The listing builds one solid part. Answer for the finished solid, in the listing's coordinates (mm). Face numbers are marked on the shaded views. Give positions to 0.01 mm unless a question says otherwise; leave off trailing zeros. Write each loop counter-clockwise with the first axis right and the second up, starting at its lowest first coordinate (ties: lowest second). Pieces come first, ordered by that corner, then holes. Notation, with made-up numbers: (27.25, -4.75) - (58.25, -4.75) arc R26 cw to (58.25, 32.25) - close; hole circle Ø2 at (68, -40). An arc over 180 degrees is marked (long way). One line per question, with ' | ' between items. Start each with the question number.
1. The mould has two halves that part along Y. Classify the marked faces 1, 2 and 3: +Y half, -Y half, draft (parallel to the pull), parting line (faces both ways), or undercut.
2. Find the intervals of material crossed by L1, parallel to Y at x = -7.15, z = 1.05; L2, parallel to X at y = 0, z = -2.9; L3, parallel to Z at x = 2, y = -1, in increasing order. Write a range as from..to.
3. A cutting plane is placed at A-A (y = 16.15). Determine the outline of the cut face in (x, z).
4. Given P1, Ø1, axis at x = 16.15, y = 0, coming from the +Z side (1 decimal); P2, Ø4.5, axis at x = -2, y = 1.5, coming from the +Z side; P3, Ø2.5, axis at x = 0, y = -7.15, coming from the +Z side; P4, Ø5, axis at x = 3, y = -12, coming from the -Z side, each flat-ended and moving along its own axis, determine where each tip first touches the part or whether it passes through.
5. A cutting plane is placed at C-C (z = -1.85). Determine the outline of the cut face in (x, y), then the cut area to 3 significant figures.
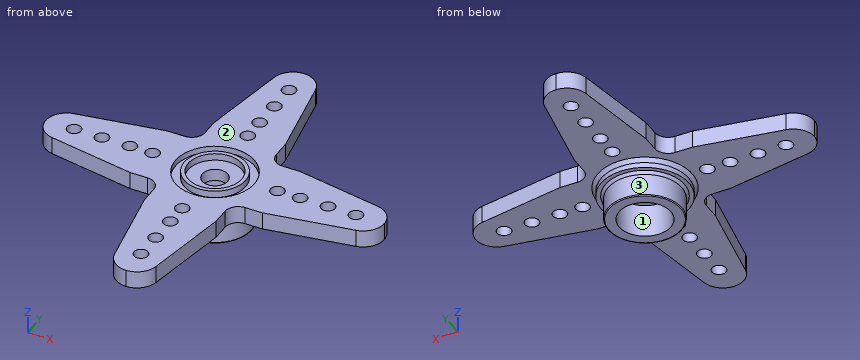
```python
from build123d import *

# Parameters (mm, degrees)
PAD_DEPTH          = 2
SKETCH001_R        = 4.5
POCKET_DEPTH       = 0.7
SKETCH002_R        = 3.5
PAD001_DEPTH       = 0.8
SKETCH003_R        = 3.05
POCKET001_DEPTH    = 0.8
SKETCH004_R        = 5
PAD002_DEPTH       = 1
SKETCH005_R        = 4.2
PAD003_DEPTH       = 2.9
SKETCH006_R        = 2.95
POCKET002_DEPTH    = 3.8
SKETCH007_R        = 1.45
POCKET003_DEPTH    = 5.201
SKETCH008_R        = 0.8
POCKET004_DEPTH    = 116.298101
POLARPATTERN_COUNT = 4
CHAMFER_SIZE       = 0.4
CHAMFER001_SIZE    = 0.3
FILLET_R           = 0.1


with BuildPart() as horn_top_left_quarter:
    # Sketch → Pad (new body)
    with BuildSketch(Plane.XY):
        with BuildLine():
            Line((0, 0), (0, 19.4))
            ThreePointArc((0, 19.4), (-1.543669, 18.837685), (-2.363981, 17.414237))
            Line((-4.086144, 7.586132), (-2.363981, 17.414237))
            Line((-4.086144, 5.586132), (-4.086144, 7.586132))
            ThreePointArc((-5.586136, 4.086144), (-4.525485, 4.525482), (-4.086144, 5.586132))
            Line((-5.586136, 4.086144), (-7.586136, 4.086144))
            Line((-17.414238, 2.363981), (-7.586136, 4.086144))
            ThreePointArc((-17.414238, 2.363981), (-18.837685, 1.543669), (-19.4, 0))
            Line((-19.4, 0), (0, 0))
        make_face()
    extrude(amount=PAD_DEPTH)


with BuildPart() as upper_half_horn:
    # Part__Mirroring: instance of horn-top-left-quarter
    add(horn_top_left_quarter.part.mirror(Plane(origin=(0, 0, 0), x_dir=(0, -1, 0), z_dir=(1, 0, 0))))

    # Fusion: union horn-top-left-quarter
    add(horn_top_left_quarter.part)


with BuildPart() as horn_final:
    # Part__Mirroring001: instance of Upper-half-horn
    add(upper_half_horn.part.mirror(Plane(origin=(0, 0, 0), x_dir=(1, 0, 0), z_dir=(0, 1, 0))))

    # Fusion001: union Upper-half-horn
    add(upper_half_horn.part)

    # Sketch001 (on Face24 of Fusion001) → Pocket (cut)
    with BuildSketch(Plane.XY.offset(2)):
        Circle(SKETCH001_R)
    extrude(amount=-POCKET_DEPTH, mode=Mode.SUBTRACT)

    # Sketch002 (on Face28 of Pocket) → Pad001 (new body)
    with BuildSketch(Plane.XY.offset(1.3)):
        Circle(SKETCH002_R)
    extrude(amount=PAD001_DEPTH)

    # Sketch003 (on Face30 of Pad001) → Pocket001 (cut)
    with BuildSketch(Plane.XY.offset(2.1)):
        Circle(SKETCH003_R)
    extrude(amount=-POCKET001_DEPTH, mode=Mode.SUBTRACT)

    # Sketch004 (on Face4 of Pocket001) → Pad002 (new body)
    with BuildSketch(Plane(origin=(0, 0, 0), x_dir=(1, 0, 0), z_dir=(0, 0, -1))):
        Circle(SKETCH004_R)
    extrude(amount=PAD002_DEPTH)

    # Sketch005 (on Face29 of Pad002) → Pad003 (new body)
    with BuildSketch(Plane(origin=(0, 0, -1), x_dir=(1, 0, 0), z_dir=(0, 0, -1))):
        Circle(SKETCH005_R)
    extrude(amount=PAD003_DEPTH)

    # Sketch006 (on Face33 of Pad003) → Pocket002 (cut)
    with BuildSketch(Plane(origin=(0, 0, -3.9), x_dir=(1, 0, 0), z_dir=(0, 0, -1))):
        Circle(SKETCH006_R)
    extrude(amount=-POCKET002_DEPTH, mode=Mode.SUBTRACT)

    # Sketch007 (on Face38 of Pocket002) → Pocket003 (cut, through all)
    with BuildSketch(Plane.XY.offset(1.3)):
        Circle(SKETCH007_R)
    extrude(amount=-POCKET003_DEPTH, mode=Mode.SUBTRACT)

    # Sketch008 (on Face5 of Pocket003) → Pocket004 (cut, through all)
    with BuildSketch(Plane.XY.offset(2)):
        with Locations((0, 16.15)):
            Circle(SKETCH008_R)
        with Locations((0, 12.95)):
            Circle(SKETCH008_R)
        with Locations((0, 9.75)):
            Circle(SKETCH008_R)
        with Locations((0, 7.15)):
            Circle(SKETCH008_R)
    pocket004 = extrude(amount=-POCKET004_DEPTH, mode=Mode.SUBTRACT)

    # PolarPattern: Pocket004 ×4 about axis
    polarpattern_axis = Axis((0, 0, 2), (0, 0, 1))
    for i in range(1, POLARPATTERN_COUNT):
        add(pocket004.rotate(polarpattern_axis, i * 360 / POLARPATTERN_COUNT), mode=Mode.SUBTRACT)

    # Chamfer
    chamfer_edges = [horn_final.edges().sort_by_distance(p)[0] for p in [
        (-5, 0, 0),
    ]]
    chamfer(chamfer_edges, length=CHAMFER_SIZE)

    # Chamfer001
    chamfer001_edges = [horn_final.edges().sort_by_distance(p)[0] for p in [
        (-4.2, 0, -1),
    ]]
    chamfer(chamfer001_edges, length=CHAMFER001_SIZE)

    # Fillet
    fillet_edges = [horn_final.edges().sort_by_distance(p)[0] for p in [
        (-4.2, 0, -3.9),
    ]]
    fillet(fillet_edges, radius=FILLET_R)


solid = horn_final.part
```
Determined:
1) face 1: undercut | face 2: draft | face 3: parting line
2) L1: -4.09..-0.8, 0.8..4.09 | L2: -4.2..-2.95, 2.95..4.2 | L3: -0.1..1.3
3) outline: (-2.59, 0) - (-0.8, 0) - (-0.8, 2) - (-2.59, 2) - close; (0.8, 0) - (2.59, 0) - (2.59, 2) - (0.8, 2) - close
4) P1: through | P2: z = 2.1 | P3: z = 2 | P4: z = 0
5) outline: circle Ø8.4 at (0, 0); hole circle Ø5.9 at (0, 0) | area: 28.1 mm2
